```python
from build123d import *

# Parameters (mm, degrees)
SHEET_EXTRUSION_DEPTH           = 3
ESQUISSE_TROU_ROUE_DROITE_W     = 70
ESQUISSE_TROU_ROUE_DROITE_H     = 40
LEFTWHEEL_EXTRUSION_DEPTH       = 219.408952171
ESQUISSE20_W                    = 30
ESQUISSE20_H                    = 17
LEFTFREEWHEEL_HOLE_DEPTH        = 219.408952171
LEFTWHEEL_FIX_OUTLINE_R         = 2.5
LEFTWHEEL_FIX_DEPTH             = 3
BALL_EXTRUSION_OUTLINE_R        = 12
BALL_EXTRUSION_DEPTH            = 3
ARROUND_FIX_EXTRUSION_OUTLINE_R = 2.5
ARROUND_FIX_EXTRUSION_DEPTH     = 3
LEFT_PROFILE_HOLE_OUTLINE_R     = 2.5
LEFT_PROFILE_HOLE_DEPTH         = 3
LEFT_FIX_MECA_SKETCH_R          = 1.5
LEFT_FIX_MECA_EXTRUSION_DEPTH   = 219.408952171
LEFT_CODER_HOLES_SKETCH_R       = 1.5
LEFT_CODER_HOLES_DEPTH          = 219.408952171
BOTTOM_FIX_HOLES_SKETCH_R       = 1.5
RIGHT_FIX_MECA_HOLES_DEPTH      = 219.408952171
SKETCH1_R                       = 1.6
BOSS_EXTRUDE1_DEPTH             = 3
BOSS_EXTRUDE2_DEPTH             = 4
SKETCH2_W                       = 3
SKETCH2_H                       = 308.847763108
CUT_EXTRUDE1_DEPTH              = 269.911228609
SKETCH3_R                       = 4.25
CUT_EXTRUDE4_DEPTH              = 209.157310334


# Read off the part's stored shape, not the designer's step: LeftWheel-Fix, Ball-Extrusion, Arround-Fix-Extrusion, Left-Profile-Hole
with BuildPart() as part:
    # Sheet-Sketch → Sheet-Extrusion (new body)
    with BuildSketch(Plane.XY):
        Polygon((-62.5, 154.423881554), (62.5, 154.423881554), (65.5, 154.423881554), (65.5, 109.423881554), (39, 75), (20, 75), (20, -75), (39, -75), (65.5, -109.423881554), (65.5, -154.423881554), (62.5, -154.423881554), (-62.5, -154.423881554), (-154.423881554, -62.5), (-154.423881554, 62.5), align=None)
    extrude(amount=SHEET_EXTRUSION_DEPTH)

    # Esquisse Trou Roue Droite → LeftWheel-Extrusion (cut, through all)
    with BuildSketch(Plane.XY.offset(3)):
        with Locations((1.237734866, 107.423881554)):
            Rectangle(ESQUISSE_TROU_ROUE_DROITE_W, ESQUISSE_TROU_ROUE_DROITE_H)
    leftwheel_extrusion = extrude(amount=-LEFTWHEEL_EXTRUSION_DEPTH, mode=Mode.SUBTRACT)

    # Esquisse20 → LeftFreeWheel-Hole (cut, through all)
    with BuildSketch(Plane.XY.offset(3)):
        with Locations((1.402864765, 135.923881554)):
            Rectangle(ESQUISSE20_W, ESQUISSE20_H)
    leftfreewheel_hole = extrude(amount=-LEFTFREEWHEEL_HOLE_DEPTH, mode=Mode.SUBTRACT)

    # LeftWheel-Fix outline → LeftWheel-Fix (cut)
    with BuildSketch(Plane.XY):
        with Locations((0.388540939, 40)):
            Circle(LEFTWHEEL_FIX_OUTLINE_R)
    leftwheel_fix = extrude(amount=LEFTWHEEL_FIX_DEPTH, mode=Mode.SUBTRACT)

    # Ball-Extrusion outline → Ball-Extrusion (cut)
    with BuildSketch(Plane.XY):
        with Locations((-114.423881554, 0)):
            Circle(BALL_EXTRUSION_OUTLINE_R)
    extrude(amount=BALL_EXTRUSION_DEPTH, mode=Mode.SUBTRACT)

    # Arround-Fix-Extrusion outline → Arround-Fix-Extrusion (cut)
    with BuildSketch(Plane.XY):
        with Locations((60.248995228, 148.862139245)):
            Circle(ARROUND_FIX_EXTRUSION_OUTLINE_R)
        with Locations((-60.248995228, 148.862139245)):
            Circle(ARROUND_FIX_EXTRUSION_OUTLINE_R)
        with Locations((-148.862139245, 60.248995228)):
            Circle(ARROUND_FIX_EXTRUSION_OUTLINE_R)
    arround_fix_extrusion = extrude(amount=ARROUND_FIX_EXTRUSION_DEPTH, mode=Mode.SUBTRACT)

    # Left-Profile-Hole outline → Left-Profile-Hole (cut)
    with BuildSketch(Plane.XY):
        with Locations((-52.5, 144.423881554)):
            Circle(LEFT_PROFILE_HOLE_OUTLINE_R)
        with Locations((52.5, 144.423881554)):
            Circle(LEFT_PROFILE_HOLE_OUTLINE_R)
    left_profile_hole = extrude(amount=LEFT_PROFILE_HOLE_DEPTH, mode=Mode.SUBTRACT)

    # Left-Fix-Meca-Sketch → Left-Fix-Meca-Extrusion (cut, through all)
    with BuildSketch(Plane.XY.offset(3)):
        with Locations((27.801900038, 82.423881554)):
            Circle(LEFT_FIX_MECA_SKETCH_R)
        with Locations((58.5, 129.423881554)):
            Circle(LEFT_FIX_MECA_SKETCH_R)
    left_fix_meca_extrusion = extrude(amount=-LEFT_FIX_MECA_EXTRUSION_DEPTH, mode=Mode.SUBTRACT)

    # Left-Coder-Holes-Sketch → Left-Coder-Holes (cut, through all)
    with BuildSketch(Plane.XY.offset(3)):
        with Locations((-28.724826295, 131.423881554)):
            Circle(LEFT_CODER_HOLES_SKETCH_R)
        with Locations((31.275173705, 131.423881554)):
            Circle(LEFT_CODER_HOLES_SKETCH_R)
    left_coder_holes = extrude(amount=-LEFT_CODER_HOLES_DEPTH, mode=Mode.SUBTRACT)

    # Bottom-Fix-Holes-Sketch → Right-Fix-Meca-Holes (cut, through all)
    with BuildSketch(Plane.XY.offset(3)):
        with Locations((-104.353414534, 105.499399209)):
            Circle(BOTTOM_FIX_HOLES_SKETCH_R)
        with Locations((-85.741045982, 80.490778132)):
            Circle(BOTTOM_FIX_HOLES_SKETCH_R)
    right_fix_meca_holes = extrude(amount=-RIGHT_FIX_MECA_HOLES_DEPTH, mode=Mode.SUBTRACT)

    # Symetry-All-Pieces: LeftWheel-Extrusion, LeftFreeWheel-Hole, LeftWheel-Fix, Arround-Fix-Extrusion, Left-Profile-Hole, Left-Fix-Meca-Extrusion, Left-Coder-Holes, Right-Fix-Meca-Holes across plane
    add(leftwheel_extrusion.mirror(Plane.ZX), mode=Mode.SUBTRACT)
    add(leftfreewheel_hole.mirror(Plane.ZX), mode=Mode.SUBTRACT)
    add(leftwheel_fix.mirror(Plane.ZX), mode=Mode.SUBTRACT)
    add(arround_fix_extrusion.mirror(Plane.ZX), mode=Mode.SUBTRACT)
    add(left_profile_hole.mirror(Plane.ZX), mode=Mode.SUBTRACT)
    add(left_fix_meca_extrusion.mirror(Plane.ZX), mode=Mode.SUBTRACT)
    add(left_coder_holes.mirror(Plane.ZX), mode=Mode.SUBTRACT)
    add(right_fix_meca_holes.mirror(Plane.ZX), mode=Mode.SUBTRACT)

    # Sketch1 → Boss-Extrude1 (add)
    with BuildSketch(Plane.XY.offset(3)):
        Polygon((-76.142135624, 140.074639149), (-69.778174593, 133.710678119), (-144.923881554, 58.564971157), (-144.923881554, -58.564971157), (-69.778174593, -133.710678119), (-76.142135624, -140.074639149), (-153.923881554, -62.292893219), (-153.923881554, 62.292893219), align=None)
        with Locations((-147.923881554, -0.5)):
            Circle(SKETCH1_R, mode=Mode.SUBTRACT)
        with Locations(Location((-103.027804769, -105.05724202, 0), (0, 0, 138.844831023))):
            Circle(SKETCH1_R, mode=Mode.SUBTRACT)
        with Locations(Location((-103.577878734, 106.274935009, 0), (0, 0, 160.535415734))):
            Circle(SKETCH1_R, mode=Mode.SUBTRACT)
    extrude(amount=BOSS_EXTRUDE1_DEPTH)

    # Sketch4 → Boss-Extrude2 (add)
    with BuildSketch(Plane.XY.offset(6)):
        Polygon((-74.02081528, 137.953318806), (-76.142135624, 140.074639149), (-153.923881554, 62.292893219), (-153.923881554, -62.292893219), (-76.142135624, -140.074639149), (-74.02081528, -137.953318806), (-150.923881554, -61.050252532), (-150.923881554, 61.050252532), align=None)
    extrude(amount=BOSS_EXTRUDE2_DEPTH)

    # Sketch2 → Cut-Extrude1 (cut, through all)
    with BuildSketch(Plane.ZY.offset(154.423881554)):
        with Locations((1.5, 0)):
            Rectangle(SKETCH2_W, SKETCH2_H)
    extrude(amount=-CUT_EXTRUDE1_DEPTH, mode=Mode.SUBTRACT)

    # Sketch3 → Cut-Extrude4 (cut, through all)
    with BuildSketch(Plane.XY.offset(6)):
        with Locations((-147.923881554, -0.5)):
            Circle(SKETCH3_R)
        with Locations((-103.577878734, 106.274935009)):
            Circle(SKETCH3_R)
        with Locations((-103.027804769, -105.05724202)):
            Circle(SKETCH3_R)
    extrude(amount=CUT_EXTRUDE4_DEPTH, mode=Mode.SUBTRACT)


solid = part.part
```
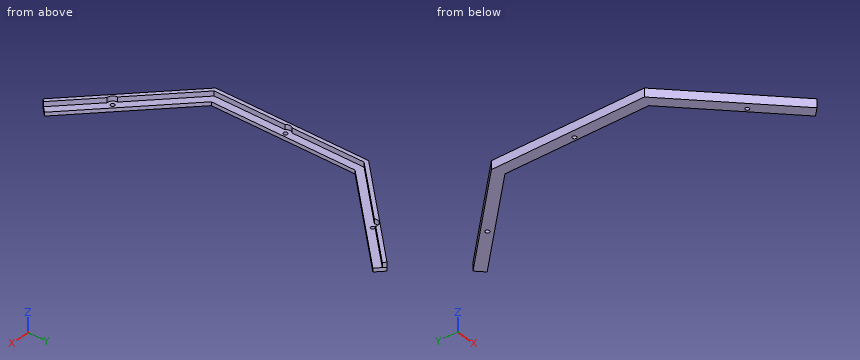
Source: CAD feature listing. Evaluate the final solid. Frame: model axes, mm. Round coordinates to 2 decimals unless told otherwise and drop trailing zeros. Loops run counter-clockwise (first coordinate to the right, second up) from the corner with the lowest first, then second, coordinate; pieces in that order, holes last.
1. Section query C-C on y = 42. Output: boundary loops of the cut face in (x, z), and give its area (3 significant figures).
2. Section query B-B on z = 7.75. Output: boundary loops of the cut face in (x, y).
3. Section query D-D on y = -94. Output: boundary loops of the cut face in (x, z), and give its area (3 significant figures).
4. Ray query, L1, parallel to Z at x = -119, y = 87; L2, parallel to Y at x = -126.5, z = 4; L3, parallel to X at y = -50, z = 8.75. Return the intervals inside material, ascending.
5. Section query A-A on x = -92.5. Output: boundary loops of the cut face in (y, z).
6. Contact query for flat-ended pins moving along their axis: pin 1 (4 mm diameter, centred on y = -22.5, z = 9, fed in from +X); pin 2 (12 mm diameter, centred on x = -103.5, y = -94, fed in from +Z); pin 3 (3 mm diameter, centred on x = -147.92, y = -0.5, fed in from +Z); pin 4 (3.5 mm diameter, centred on y = -12.5, z = 4, fed in from +X). Output: stop coordinate, or through.
Answers below:
1. outline: (-153.92, 3) - (-144.92, 3) - (-144.92, 6) - (-150.92, 6) - (-150.92, 10) - (-153.92, 10) - close
1. area: 39.0 mm2
2. outline: (-153.92, -62.29) - (-76.14, -140.07) - (-74.02, -137.95) - (-102.68, -109.29) arc R4.25 cw to (-107.26, -104.71) - (-150.92, -61.05) - (-150.92, -3.51) arc R4.25 cw to (-150.92, 2.51) - (-150.92, 61.05) - (-107.45, 104.52) arc R4.25 cw to (-101.83, 110.15) - (-74.02, 137.95) - (-76.14, 140.07) - (-153.92, 62.29) - close
3. outline: (-122.22, 3) - (-109.49, 3) - (-109.49, 6) - (-117.97, 6) - (-117.97, 10) - (-122.22, 10) - close
3. area: 55.2 mm2
4. L1: z = 3 to 6
4. L2: y = -89.72 to -76.99, 76.99 to 89.72
4. L3: x = -153.92 to -150.92
5. outline: (-123.72, 3) - (-110.99, 3) - (-110.99, 6) - (-119.47, 6) - (-119.47, 10) - (-123.72, 10) - close; (110.99, 3) - (123.72, 3) - (123.72, 10) - (119.47, 10) - (119.47, 6) - (110.99, 6) - close
6. pin 1: stops at x = -150.92
6. pin 2: stops at z = 6
6. pin 3: passes through
6. pin 4: stops at x = -144.92
